For this review, take the finished solid that the model builds, in its own axes (mm). A direction names the side the tool comes from. Round coordinates to 2 decimals unless told otherwise and drop trailing zeros. Write each loop counter-clockwise with the first axis right and the second up, starting at its lowest first coordinate (ties: lowest second). Pieces come first, ordered by that corner, then holes. Notation, with made-up numbers: (47, 87) -> (51, 87) arc R16 cw to (51, 110) -> close; hole circle Ø2 at (22.25, 11). An arc over 180 degrees is marked (long way). Answer as CSV lines item,"result". Start each with the question number.
Item 1: Wall thickness on probe 1 along Y at (x, z) = (0, 33); probe 2 along X at (y, z) = (11, 0); probe 3 along Z at (x, y) = (1, 7.5): over which ranges is each line inside the solid? List them lowest first. Write a range as from..to.
Item 2: Take a section at A-A on x = -17.5. Give the boundary of the cut face in (y, z), then the cut area to 3 significant figures.
Item 3: For pin 1 Ø7 at (x, z) = (-12.5, 0) entering from +Y; pin 2 Ø8 at (x, z) = (-14.5, 15.5) entering from -Y; pin 3 Ø6 at (x, y) = (-12.5, 25.5) entering from -Z; pin 4 Ø2.5 at (x, y) = (0, 55) entering from -Z, all flat-tipped, find the tip position at first contact; note any pin that passes through.
Item 4: Mouldability with a two-part tool opening along Z and no side actions: class faces 1 (the cylindrical face through (33.71, 56.43, -0.45)), 2 (the cylindrical face through (-28, 30, -21)), 3 (the cylindrical face through (-1.2, 54.1, -33.7)) as +Z half, -Z half, draft (parallel to the pull), parting line (faces both ways), or undercut.
Item 5: Take a section at D-D on x = 9.5. Give the boundary of the cut face in (y, z), then the cut area to 3 significant figures.
Item 6: Take a section at B-B on z = -17. Give the boundary of the cut face in (x, y).
Item 7: Machinability: for faces 4 (the flat face through (0, 30, 0)), 5 (the flat face through (0, 25, 0)), 6 (the cylindrical face through (-1.2, 55.9, 33.7)), which of the approach directions +Z, -Z, +X, -X, +Y, -Y give a long, thin tool a straight path to every point of the face, cutting with its end or side? Answer none if there is none.
Item 8: Take a section at C-C on y = 55. Give the boundary of the cut face in (x, z), then the cut area to 3 significant figures.
Autodesk Inventor part; units mm, degrees
ref_plane "YZ Plane" through (0, 0, 0) normal (1, 0, 0) x (0, 1, 0)
ref_plane "XZ Plane" through (0, 0, 0) normal (0, 1, 0) x (-1, 0, 0)
ref_plane "XY Plane" through (0, 0, 0) normal (0, 0, 1) x (1, 0, 0)
sketch "Sketch1" plane through (0, 0, 0) normal (0, 0, 1) x (1, 0, 0)
  line L0 (0, 0) -> (0, 25)
  line L1 (0, 60) -> (35, 60)
  line L2 (35, 60) -> (35, 0)
  line L3 (35, 0) -> (30, 0)
  line L4 (35, 0) -> (0, 35)
  line L5 (35, 0) -> (30, 0)
  line L6 (30, 0) -> (30, 5)
  line L7 (30, 5) -> (32.5, 5)
  line L8 (35, 5) -> (35, 0)
  line L9 (30, 5) -> (25, 5)
  line L10 (25, 5) -> (25, 10)
  line L11 (25, 10) -> (30, 10)
  line L12 (30, 10) -> (30, 5)
  line L13 (25, 10) -> (20, 10)
  line L14 (20, 10) -> (20, 15)
  line L15 (20, 15) -> (25, 15)
  line L16 (25, 15) -> (25, 10)
  line L17 (20, 15) -> (15, 15)
  line L18 (15, 15) -> (15, 20)
  line L19 (15, 20) -> (20, 20)
  line L20 (20, 20) -> (20, 15)
  line L21 (15, 20) -> (10, 20)
  line L22 (10, 20) -> (10, 25)
  line L23 (10, 25) -> (15, 25)
  line L24 (15, 25) -> (15, 20)
  line L25 (10, 25) -> (0, 25)
  line L26 (0, 25) -> (0, 60)
  line L27 (30, 0) -> (0, 0)
  line L28 (32.5, 60) -> (32.5, 0)
  line L29 (32.5, 5) -> (35, 5)
  line L30 (27.5, 10) -> (32.5, 10)
  line L31 (0, 30) -> (10, 30)
  line L32 (10, 30) -> (32.5, 30)
  point P0 (5, 30)
  point P1 (32.5, 0)
  dimension "d0" = 60
  dimension "d1" = 35
  dimension "d2" = 45
  dimension "d3" = 5
  dimension "d4" = 5
  dimension "d5" = 5
  dimension "d6" = 5
  dimension "d7" = 5
  dimension "d8" = 2.5
  dimension "d9" = 5
revolve "Revolution1" add sketch "Sketch1" angle 360 about axis through (0, 25, 0) along (0, 1, 0) contours L26 L31 L4 L25 | L4 L31 L32 L28 L30 L11 L16 L15 L20 L19 L24 L23 | L28 L4 L3 | L4 L28 L29 L2 | L28 L1 L2 L29
sketch "Sketch4" plane through (0, 10, 0) normal (0, -1, 0) x (1, 0, 0)
  circle A0 centre (0, 0) radius 32.5
  circle A1 centre (0, 0) radius 25
  line L0 (-32.5, 0) -> (-25, 0)
  point P0 (-28.75, 0)
sketch "Sketch5" plane through (0, 15, 0) normal (0, -1, 0) x (1, 0, 0)
  circle A0 centre (0, 0) radius 25
  circle A1 centre (0, 0) radius 20
  line L0 (-25, 0) -> (-20, 0)
  point P0 (-22.5, 0)
sketch "Sketch6" plane through (0, 20, 0) normal (0, -1, 0) x (1, 0, 0)
  circle A0 centre (0, 0) radius 20
  circle A1 centre (0, 0) radius 15
  line L0 (-20, 0) -> (-15, 0)
  point P0 (-17.5, 0)
sketch "Sketch7" plane through (0, 25, 0) normal (0, -1, 0) x (1, 0, 0)
  circle A0 centre (0, 0) radius 15
  line L0 (-15, 0) -> (-12.5, 0)
  dimension "d19" = 2.5
hole "Hole2" at (-28.75, 10, 0) direction (0, 1, 0) diameter 3 end through all counterbore diameter 4.5 counterbore depth 3
hole "Hole3" at (-22.5, 15, 0) direction (0, 1, 0) diameter 3 end through all counterbore diameter 4 counterbore depth 3
hole "Hole4" at (-17.5, 20, 0) direction (0, 1, 0) diameter 3 end through all counterbore diameter 4.5 counterbore depth 3
hole "Hole5" at (-12.5, 25, 0) direction (0, 1, 0) diameter 3 end through all counterbore diameter 4.5 counterbore depth 3
sketch "Sketch8" plane through (0, 0, 0) normal (0, 0, 1) x (1, 0, 0)
  line L0 (35, 60) -> (-35, 60)
  line L1 (35, 0) -> (-35, 0)
  line L2 (32.5, 60) -> (-32.5, 60)
  line L3 (0, 60) -> (0, 55)
  circle A0 centre (0, 55) radius 1.5
  point P0 (0, 0)
  dimension "d48" = 5
  dimension "d49" = 3
extrude "Extrusion1" cut sketch "Sketch8" along normal through all both and the other way through all
sketch "Sketch9" plane through (0, 0, 0) normal (1, 0, 0) x (0, 1, 0)
  line L0 (60, -35) -> (60, 35)
  line L1 (0, -35) -> (0, 35)
  line L2 (60, 0) -> (55, 0)
  circle A0 centre (55, 0) radius 1.5
  point P0 (0, 0)
  point P1 (55, 34.9678)
  point P2 (55, -34.9678)
  dimension "d52" = 5
  dimension "d53" = 3
extrude "Extrusion2" cut sketch "Sketch9" along normal through all both and the other way through all
properties part number "Grundkörper"
Output values:
1,probe 1,"y = 0..53.5, 56.5..60"
1,probe 2,"x = -35..-31, -26.5..-25, 25..35"
1,probe 3,"z = -34.99..-32.48, 32.48..34.99"
2,outline,"(0, -30.31) -> (60, -30.31) -> (60, -27.39) -> (30, -27.39) -> (30, -1.5) -> (23, -1.5) -> (23, -2.25) -> (20, -2.25) -> (20, -9.68) -> (15, -9.68) -> (15, -17.85) -> (10, -17.85) -> (10, -27.39) -> (0, -27.39) -> close; (0, 27.39) -> (10, 27.39) -> (10, 17.85) -> (15, 17.85) -> (15, 9.68) -> (20, 9.68) -> (20, 2.25) -> (23, 2.25) -> (23, 1.5) -> (30, 1.5) -> (30, 27.39) -> (60, 27.39) -> (60, 30.31) -> (0, 30.31) -> close"
2,area,"1,140 mm^2"
3,pin 1,"stops at y = 30"
3,pin 2,"stops at y = 10"
3,pin 3,"stops at z = -33.69"
3,pin 4,"passes through"
4,face 1,"undercut"
4,face 2,"parting line"
4,face 3,"draft"
5,outline,"(0, -33.69) -> (60, -33.69) -> (60, -31.08) -> (30, -31.08) -> (30, 31.08) -> (60, 31.08) -> (60, 33.69) -> (0, 33.69) -> (0, 31.08) -> (10, 31.08) -> (10, 23.12) -> (15, 23.12) -> (15, 17.6) -> (20, 17.6) -> (20, 11.61) -> (25, 11.61) -> (25, -11.61) -> (20, -11.61) -> (20, -17.6) -> (15, -17.6) -> (15, -23.12) -> (10, -23.12) -> (10, -31.08) -> (0, -31.08) -> close"
5,area,"1,030 mm^2"
6,outline,"(-30.59, 0) -> (-27.7, 0) -> (-27.7, 10) -> (-18.33, 10) -> (-18.33, 15) -> (-10.54, 15) -> (-10.54, 20) -> (10.54, 20) -> (10.54, 15) -> (18.33, 15) -> (18.33, 10) -> (27.7, 10) -> (27.7, 0) -> (30.59, 0) -> (30.59, 60) -> (27.7, 60) -> (27.7, 30) -> (-27.7, 30) -> (-27.7, 60) -> (-30.59, 60) -> close"
7,face 4,"+Y"
7,face 5,"-Y"
7,face 6,"+Z, -Z"
8,outline,"(-34.97, -1.5) arc R35 ccw to (-1.5, -34.97) -> (-1.5, -32.47) arc R32.5 cw to (-32.47, -1.5) -> close; (-34.97, 1.5) -> (-32.47, 1.5) arc R32.5 cw to (-1.5, 32.47) -> (-1.5, 34.97) arc R35 ccw to start; (1.5, -34.97) arc R35 ccw to (34.97, -1.5) -> (32.47, -1.5) arc R32.5 cw to (1.5, -32.47) -> close; (1.5, 32.47) arc R32.5 cw to (32.47, 1.5) -> (34.97, 1.5) arc R35 ccw to (1.5, 34.97) -> close"
8,area,"500 mm^2"
